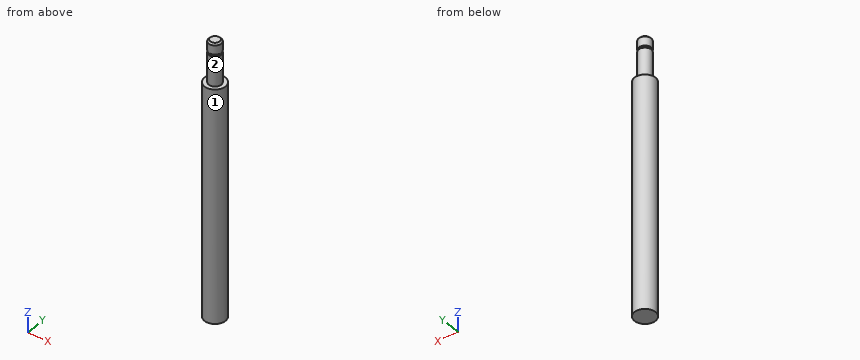
```python
from build123d import *

# Parameters (mm, degrees)
SKETCH_1_R          = 10
EXTRUDE_1_DEPTH     = 260
SKETCH_2_OUTSIDE_W  = 74.306
SKETCH_2_OUTSIDE_H  = 74.306
SKETCH_2_OUTSIDE_R  = 6
CUT_EXTRUDE_1_DEPTH = 40
SKETCH_3_OUTSIDE_W  = 74.306
SKETCH_3_OUTSIDE_H  = 74.306
SKETCH_3_OUTSIDE_R  = 5
CUT_EXTRUDE_2_DEPTH = 2
CHAMFER_1_SIZE      = 1.5


with BuildPart() as part:
    # 草图1 → 凸台-拉伸1 (new body)
    with BuildSketch(Plane.XY):
        Circle(SKETCH_1_R)
    extrude(amount=EXTRUDE_1_DEPTH)

    # 草图2 outside → 切除-拉伸1 (cut)
    with BuildSketch(Plane.XY.offset(260)):
        Rectangle(SKETCH_2_OUTSIDE_W, SKETCH_2_OUTSIDE_H)
        Circle(SKETCH_2_OUTSIDE_R, mode=Mode.SUBTRACT)
    extrude(amount=-CUT_EXTRUDE_1_DEPTH, mode=Mode.SUBTRACT)

    # 草图3 outside → 切除-拉伸2 (cut)
    with BuildSketch(Plane.XY.offset(250)):
        Rectangle(SKETCH_3_OUTSIDE_W, SKETCH_3_OUTSIDE_H)
        Circle(SKETCH_3_OUTSIDE_R, mode=Mode.SUBTRACT)
    extrude(amount=-CUT_EXTRUDE_2_DEPTH, mode=Mode.SUBTRACT)

    # 倒角1
    chamfer_1_edges = [part.edges().sort_by_distance(p)[0] for p in [
        (-6, 0, 260),
    ]]
    chamfer(chamfer_1_edges, length=CHAMFER_1_SIZE)


solid = part.part
```
Can you work these out from the model? Positions are in its coordinate system, mm. Face numbers are marked on the shaded views. A direction names the side the tool comes from. Give positions to 0.01 mm unless a question says otherwise; leave off trailing zeros. Write each loop counter-clockwise with the first axis right and the second up, starting at its lowest first coordinate (ties: lowest second). Pieces come first, ordered by that corner, then holes. Notation, with made-up numbers: (21, -14) - (39, -14) arc R13 cw to (39, -10) - close; hole circle Ø5 at (41.5, -8). An arc over 180 degrees is marked (long way). Write item = value, one per line. Start each with the question number.
1. Imagine slicing it at A-A (y = 0). Please give me the cut outline in (x, z), and give its area (3 significant figures).
2. For pin 1 (2 mm diameter, centred on y = 6, z = 74, fed in from -X); pin 2 (1.5 mm diameter, centred on x = -3.5, z = 233.5, fed in from -Y); pin 3 (6 mm diameter, centred on x = -5, z = 168.5, fed in from -Y), each with a flat end and sliding along its axis, tell me the tip position at first contact or that it passes through.
3. On a 3-axis mill with a long thin cutter (end or side, diameter ignored), from which of +Z, -Z, +X, -X, +Y, -Y can I reach the whole of each face in a straight line? I mean the marked faces 1 and 2. Say none if no direction works.
4. Imagine slicing it at D-D (z = 240.5). Please give me the cut outline in (x, y), and give its area (3 significant figures).
5. Imagine slicing it at C-C (z = 106). Please give me the cut outline in (x, y), and give its area (3 significant figures).
6. Please list where these lines run through material, in increasing order: line 1 (X direction, y = -8, z = 57.5); line 2 (Z direction, x = 1.75, y = -6.25); line 3 (Y direction, x = 0.75, z = 144.5).
Worked answers:
q1.outline = (-10, 0) - (10, 0) - (10, 220) - (6, 220) - (6, 248) - (5, 248) - (5, 250) - (6, 250) - (6, 258.5) - (4.5, 260) - (-4.5, 260) - (-6, 258.5) - (-6, 250) - (-5, 250) - (-5, 248) - (-6, 248) - (-6, 220) - (-10, 220) - close
q1.area = 4,870 mm2
q2.pin_1 = -8.66
q2.pin_2 = -5.33
q2.pin_3 = -9.8
q3.face_1 = +Z, -Z
q3.face_2 = +Z
q4.outline = circle Ø12 at (0, 0)
q4.area = 113 mm2
q5.outline = circle Ø20 at (0, 0)
q5.area = 314 mm2
q6.line_1 = -6 to 6
q6.line_2 = 0 to 220
q6.line_3 = -9.97 to 9.97
